The listing builds one solid part. Answer for the finished solid, in the listing's coordinates (mm). Round coordinates to 2 decimals unless told otherwise and drop trailing zeros. Answer as a JSON object with one key per item and string values.
```python
from build123d import *

# Parameters (mm, degrees)
SKETCH4_W              = 20
SKETCH4_H              = 20
BODY_DEPTH             = 240
SKETCH16_OUTSIDE_W     = 70.332
SKETCH16_OUTSIDE_H     = 70.332
SKETCH16_OUTSIDE_R     = 2.15
CUT_PROFILE_DEPTH      = 26
CUT_PROFILE_DEPTH_BACK = 216


with BuildPart() as part:
    # Sketch4 → Body (new body)
    with BuildSketch(Plane.XY.offset(25)):
        Rectangle(SKETCH4_W, SKETCH4_H)
    extrude(amount=-BODY_DEPTH)

    # Sketch16 outside → Cut-Profile (cut, two sides)
    with BuildSketch(Plane.XY) as cut_profile_sk:
        Rectangle(SKETCH16_OUTSIDE_W, SKETCH16_OUTSIDE_H)
        with BuildLine():
            Line((4.917588389, -8.199999991), (2.799999989, -8.199999991))
            ThreePointArc((2.799999989, -8.199999991), (2.587867955, -8.287867957), (2.499999989, -8.499999991))
            Line((2.499999989, -8.499999991), (2.499999989, -9.199999991))
            ThreePointArc((2.499999989, -9.199999991), (2.734314564, -9.765685416), (3.299999989, -9.999999991))
            Line((3.299999989, -9.999999991), (7.999999989, -9.999999991))
            ThreePointArc((7.999999989, -9.999999991), (9.414213552, -9.414213554), (9.999999989, -7.999999991))
            Line((9.999999989, -7.999999991), (9.999999989, -3.299999991))
            ThreePointArc((9.999999989, -3.299999991), (9.765685414, -2.734314566), (9.199999989, -2.499999991))
            Line((9.199999989, -2.499999991), (8.499999989, -2.499999991))
            ThreePointArc((8.499999989, -2.499999991), (8.287867955, -2.587867957), (8.199999989, -2.799999991))
            Line((8.199999989, -2.799999991), (8.199999989, -4.917588391))
            ThreePointArc((8.199999989, -4.917588391), (7.686138511, -5.686636441), (6.778984485, -5.506192286))
            Line((6.778984485, -5.506192286), (4.528679645, -3.255887446))
            ThreePointArc((4.528679645, -3.255887446), (3.878361392, -2.282617401), (3.64999999, -1.134567106))
            Line((3.64999999, -1.134567106), (3.64999999, 1.134567104))
            ThreePointArc((3.64999999, 1.134567104), (3.878361393, 2.282617402), (4.528679647, 3.255887448))
            Line((4.528679647, 3.255887448), (6.778984487, 5.506192288))
            ThreePointArc((6.778984487, 5.506192288), (7.686138506, 5.686636442), (8.199999981, 4.917588398))
            Line((8.199999981, 4.917588398), (8.199999981, 2.799999998))
            ThreePointArc((8.199999981, 2.799999998), (8.287867946, 2.587867964), (8.499999981, 2.499999998))
            Line((8.499999981, 2.499999998), (9.199999981, 2.499999998))
            ThreePointArc((9.199999981, 2.499999998), (9.765685406, 2.734314573), (9.999999981, 3.299999998))
            Line((9.999999981, 3.299999998), (9.999999981, 7.999999998))
            ThreePointArc((9.999999981, 7.999999998), (9.414213543, 9.41421356), (7.999999981, 9.999999998))
            Line((7.999999981, 9.999999998), (3.299999981, 9.999999998))
            ThreePointArc((3.299999981, 9.999999998), (2.734314556, 9.765685423), (2.499999981, 9.199999998))
            Line((2.499999981, 9.199999998), (2.499999981, 8.499999998))
            ThreePointArc((2.499999981, 8.499999998), (2.587867946, 8.287867964), (2.799999981, 8.199999998))
            Line((2.799999981, 8.199999998), (4.917588381, 8.199999998))
            ThreePointArc((4.917588381, 8.199999998), (5.68663643, 7.68613852), (5.506192275, 6.778984494))
            Line((5.506192275, 6.778984494), (3.255887435, 4.528679654))
            ThreePointArc((3.255887435, 4.528679654), (2.28261739, 3.878361401), (1.134567095, 3.649999999))
            Line((1.134567095, 3.649999999), (-1.134567115, 3.649999999))
            ThreePointArc((-1.134567115, 3.649999999), (-2.282617412, 3.878361401), (-3.255887459, 4.528679655))
            Line((-3.255887459, 4.528679655), (-5.506192299, 6.778984495))
            ThreePointArc((-5.506192299, 6.778984495), (-5.686636452, 7.686138515), (-4.917588409, 8.199999989))
            Line((-4.917588409, 8.199999989), (-2.800000009, 8.199999989))
            ThreePointArc((-2.800000009, 8.199999989), (-2.587867974, 8.287867955), (-2.500000009, 8.499999989))
            Line((-2.500000009, 8.499999989), (-2.500000009, 9.199999989))
            ThreePointArc((-2.500000009, 9.199999989), (-2.734314584, 9.765685414), (-3.300000009, 9.999999989))
            Line((-3.300000009, 9.999999989), (-8.000000009, 9.999999989))
            ThreePointArc((-8.000000009, 9.999999989), (-9.414213571, 9.414213552), (-10.000000009, 7.999999989))
            Line((-10.000000009, 7.999999989), (-10.000000009, 3.299999989))
            ThreePointArc((-10.000000009, 3.299999989), (-9.765685434, 2.734314564), (-9.200000009, 2.499999989))
            Line((-9.200000009, 2.499999989), (-8.500000009, 2.499999989))
            ThreePointArc((-8.500000009, 2.499999989), (-8.287867974, 2.587867955), (-8.200000009, 2.799999989))
            Line((-8.200000009, 2.799999989), (-8.200000009, 4.917588389))
            ThreePointArc((-8.200000009, 4.917588389), (-7.686138531, 5.686636438), (-6.778984504, 5.506192284))
            Line((-6.778984504, 5.506192284), (-4.528679664, 3.255887444))
            ThreePointArc((-4.528679664, 3.255887444), (-3.878361412, 2.282617399), (-3.650000009, 1.134567104))
            Line((-3.650000009, 1.134567104), (-3.650000009, -1.134567106))
            ThreePointArc((-3.650000009, -1.134567106), (-3.878361412, -2.282617404), (-4.528679666, -3.25588745))
            Line((-4.528679666, -3.25588745), (-6.778984506, -5.50619229))
            ThreePointArc((-6.778984506, -5.50619229), (-7.686138526, -5.686636444), (-8.2, -4.9175884))
            Line((-8.2, -4.9175884), (-8.2, -2.8))
            ThreePointArc((-8.2, -2.8), (-8.287867966, -2.587867966), (-8.5, -2.5))
            Line((-8.5, -2.5), (-9.2, -2.5))
            ThreePointArc((-9.2, -2.5), (-9.765685425, -2.734314575), (-10, -3.3))
            Line((-10, -3.3), (-10, -8))
            ThreePointArc((-10, -8), (-9.414213562, -9.414213562), (-8, -10))
            Line((-8, -10), (-3.3, -10))
            ThreePointArc((-3.3, -10), (-2.734314575, -9.765685425), (-2.5, -9.2))
            Line((-2.5, -9.2), (-2.5, -8.5))
            ThreePointArc((-2.5, -8.5), (-2.587867966, -8.287867966), (-2.8, -8.2))
            Line((-2.8, -8.2), (-4.9175884, -8.2))
            ThreePointArc((-4.9175884, -8.2), (-5.686636449, -7.686138522), (-5.506192294, -6.778984496))
            Line((-5.506192294, -6.778984496), (-3.255887454, -4.528679656))
            ThreePointArc((-3.255887454, -4.528679656), (-2.282617409, -3.878361403), (-1.134567114, -3.650000001))
            Line((-1.134567114, -3.650000001), (1.134567096, -3.650000001))
            ThreePointArc((1.134567096, -3.650000001), (2.282617393, -3.878361403), (3.255887439, -4.528679657))
            Line((3.255887439, -4.528679657), (5.506192279, -6.778984497))
            ThreePointArc((5.506192279, -6.778984497), (5.686636433, -7.686138517), (4.917588389, -8.199999991))
        make_face(mode=Mode.SUBTRACT)
        Circle(SKETCH16_OUTSIDE_R)
    extrude(amount=CUT_PROFILE_DEPTH, mode=Mode.SUBTRACT)
    extrude(cut_profile_sk.sketch, amount=-CUT_PROFILE_DEPTH_BACK, mode=Mode.SUBTRACT)


solid = part.part
```
Item 1: Flat-ended cylindrical pins translate along their axes: P1, Ø0.6, axis at x = -9, z = -41.5, coming from the -Y side; P2, Ø1.8, axis at x = 0, z = -125, coming from the -Y side; P3, Ø0.6, axis at y = -9, z = -64, coming from the -X side. Find the tip coordinate at first contact, or state that the pin passes through.
Values follow:
{"P1": "y = -9.87", "P2": "y = -3.65", "P3": "x = -9.87"}
Item 2: Straight lines are drawn through the part: line 1 (Y direction, x = 0, z = -157.5); line 2 (X direction, y = -4.75, z = -173). For each, find the intervals that lie inside material, in ascending order.
Values follow:
{"line 1": "-3.65 to -2.15, 2.15 to 3.65", "line 2": "-10 to -8.2, -6.02 to -3.48, 3.48 to 6.02, 8.2 to 10"}
Item 3: Determine the mould class of faces 1 (the face through (-2.15, 0.09, -93.32)), 2 (the face through (10, 6, -93)), 3 (the face through (6, 10, -93)) for opening direction X: released by +X, released by -X, zero draft, split by the parting line, or undercut.
Values follow:
{"face 1": "undercut", "face 2": "released by +X", "face 3": "zero draft"}
